```python
from build123d import *

# Parameters (mm, degrees)
F1_DEPTH = 19.05


with BuildPart() as f1:
    # F0 (on Top) → F1 (new body)
    with BuildSketch(Plane.XY):
        with BuildLine():
            Line((895.35, 0), (0, 0))
            Line((0, 0), (0, -552.45))
            Line((0, -552.45), (3.175, -552.45))
            ThreePointArc((3.175, -552.45), (7.665128, -554.309872), (9.525, -558.8))
            Line((9.525, -558.8), (9.525, -590.55))
            Line((9.525, -590.55), (885.825, -590.55))
            Line((885.825, -590.55), (885.825, -558.8))
            ThreePointArc((885.825, -558.8), (887.684872, -554.309872), (892.175, -552.45))
            Line((892.175, -552.45), (895.35, -552.45))
            Line((895.35, -552.45), (895.35, 0))
        make_face()
    extrude(amount=F1_DEPTH)


solid = f1.part
```
Could you check a few things on this model? Use its own coordinates, in mm. A direction names the side the tool comes from. Round coordinates to 2 decimals unless told otherwise and drop trailing zeros. One line per question, with ' | ' between items.
(1) If I drill on probe 1 along X at (y, z) = (-564, 2.5) (3 decimals), over which ranges is the centre line in solid material (lowest first)?
Model answer:
probe 1: x = 9.525 to 885.825
(2) For faces 1 (the face through (441, -291, 19.05)), 2 (the face through (885.825, -575, 9)), 3 (the face through (9.525, -574, 9)), which set-ups out of +Z, -Z, +X, -X, +Y, -Y let a thin tool reach every point of the face, with its end or its side?
Model answer:
face 1: +Z, +X, -X, +Y, -Y | face 2: +Z, -Z, +X, -Y | face 3: +Z, -Z, -X, -Y
(3) For pin 1 Ø9.5 at (y, z) = (-569, 12.5) entering from +X (3 decimals); pin 2 Ø1 at (x, z) = (893, 5) entering from -Y; pin 3 Ø5.5 at (y, z) = (-570.5, 12.5) entering from -X (3 decimals), each with a flat end and sliding along its axis, tell me the tip position at first contact or that it passes through.
Model answer:
pin 1: stops at x = 885.825 | pin 2: stops at y = -552.45 | pin 3: stops at x = 9.525
